Source: CAD feature listing. Evaluate the final solid. Frame: model axes, mm. A direction names the side the tool comes from. Round coordinates to 2 decimals unless told otherwise and drop trailing zeros. Order: outer loops, then holes, each group sorted by start corner. A loop starts at its lowest first (then second) coordinate and runs counter-clockwise, first axis right, second up. Notation, with made-up numbers: M 55.25,-4.75 L 78.25,-4.75 A24 ccw 78.25,29.25 Z; hole C -14,-18.75 d5. An arc over 180 degrees is marked long. Answer in a Markdown table with one row per item. Add a question column.
```python
from build123d import *

# Parameters (mm, degrees)
SKETCH1_W                 = 123
SKETCH1_H                 = 87.75
SKETCH1_W_2               = 113
SKETCH1_H_2               = 77.75
BOSS_EXTRUDE1_DEPTH       = 44
SKETCH1_3_W               = 113
SKETCH1_3_H               = 77.75
BOSS_EXTRUDE2_DEPTH       = 3
FILLET1_R                 = 15
FILLET2_R                 = 15
FILLET3_R                 = 15
FILLET4_R                 = 15
FILLET5_R                 = 15
FILLET6_R                 = 15
FILLET7_R                 = 15
FILLET8_R                 = 15
SKETCH2_R                 = 1.5
CUT_EXTRUDE1_DEPTH        = 116.837439975
LPATTERN2_COUNT           = 2
LPATTERN2_PITCH           = 32
LPATTERN2_COPY_1_SKETCH_R = 1.5
LPATTERN2_COPY_1_DEPTH    = 116.837439975
SKETCH3_R                 = 12.5
CUT_EXTRUDE2_DEPTH        = 138.804265627


with BuildPart() as part:
    # Sketch1 → Boss-Extrude1 (new body)
    with BuildSketch(Plane(origin=(0, 0, 0), x_dir=(1, 0, 0), z_dir=(0, 1, 0))):
        Rectangle(SKETCH1_W, SKETCH1_H)
        Rectangle(SKETCH1_W_2, SKETCH1_H_2, mode=Mode.SUBTRACT)
    extrude(amount=BOSS_EXTRUDE1_DEPTH)

    # Sketch1_3 → Boss-Extrude2 (add)
    with BuildSketch(Plane(origin=(0, 0, 0), x_dir=(1, 0, 0), z_dir=(0, 1, 0))):
        Rectangle(SKETCH1_3_W, SKETCH1_3_H)
    extrude(amount=BOSS_EXTRUDE2_DEPTH)

    # Fillet1
    fillet1_edges = [part.edges().sort_by_distance(p)[0] for p in [
        (-61.5, 22, 43.875),
    ]]
    fillet(fillet1_edges, radius=FILLET1_R)

    # Fillet2
    fillet2_edges = [part.edges().sort_by_distance(p)[0] for p in [
        (-61.5, 22, -43.875),
    ]]
    fillet(fillet2_edges, radius=FILLET2_R)

    # Fillet3
    fillet3_edges = [part.edges().sort_by_distance(p)[0] for p in [
        (61.5, 22, -43.875),
    ]]
    fillet(fillet3_edges, radius=FILLET3_R)

    # Fillet4
    fillet4_edges = [part.edges().sort_by_distance(p)[0] for p in [
        (61.5, 22, 43.875),
    ]]
    fillet(fillet4_edges, radius=FILLET4_R)

    # Fillet5
    fillet5_edges = [part.edges().sort_by_distance(p)[0] for p in [
        (-56.5, 23.5, -38.875),
    ]]
    fillet(fillet5_edges, radius=FILLET5_R)

    # Fillet6
    fillet6_edges = [part.edges().sort_by_distance(p)[0] for p in [
        (-56.5, 23.5, 38.875),
    ]]
    fillet(fillet6_edges, radius=FILLET6_R)

    # Fillet7
    fillet7_edges = [part.edges().sort_by_distance(p)[0] for p in [
        (56.5, 23.5, -38.875),
    ]]
    fillet(fillet7_edges, radius=FILLET7_R)

    # Fillet8
    fillet8_edges = [part.edges().sort_by_distance(p)[0] for p in [
        (56.5, 23.5, 38.875),
    ]]
    fillet(fillet8_edges, radius=FILLET8_R)

    # Sketch2 → Cut-Extrude1 (cut, through all)
    with BuildSketch(Plane(origin=(0, 0, -43.875), x_dir=(-1, 0, 0), z_dir=(0, 0, -1))):
        with Locations((-25.75, 6.25)):
            Circle(SKETCH2_R)
    cut_extrude1 = extrude(amount=-CUT_EXTRUDE1_DEPTH, mode=Mode.SUBTRACT)

    # Mirror1: Cut-Extrude1 across plane
    add(cut_extrude1.mirror(Plane(origin=(0, 0, 0), x_dir=(0, 0, 1), z_dir=(1, 0, 0))), mode=Mode.SUBTRACT)

    # LPattern2: Cut-Extrude1 ×2
    with Locations(*[(0, i * LPATTERN2_PITCH, 0) for i in range(1, LPATTERN2_COUNT)]):
        add(cut_extrude1, mode=Mode.SUBTRACT)

    # LPattern2 copy 1 sketch → LPattern2 copy 1 (cut, through all)
    with BuildSketch(Plane(origin=(0, 32, -43.875), x_dir=(1, 0, 0), z_dir=(0, 0, -1))):
        with Locations((-25.75, -6.25)):
            Circle(LPATTERN2_COPY_1_SKETCH_R)
    extrude(amount=-LPATTERN2_COPY_1_DEPTH, mode=Mode.SUBTRACT)

    # Sketch3 → Cut-Extrude2 (cut, through all)
    with BuildSketch(Plane.ZY.offset(61.5)):
        with Locations((0, 23.62)):
            Circle(SKETCH3_R)
    extrude(amount=-CUT_EXTRUDE2_DEPTH, mode=Mode.SUBTRACT)


solid = part.part
```
(1) Pin query (flat end, axial travel): pin 1 (1.5 mm diameter, centred on x = -24.5, z = 0.5, fed in from +Y). Return the tip coordinate at first contact, or that it passes through.
(2) Access query for faces 5 (the face through (56.989, 22.308, -39.598)), 6 (the face through (-1, 3, -1)). Directions: +Z, -Z, +X, -X, +Y, -Y. A direction counts if a zero-diameter tool reaches every point of the face in a straight line with its end or side. Return the directions, or none.
(3) Cut plane D-D (x = -4). Return loops of the section in (y, z) (3 decimals), and give its area (3 significant figures).
(4) Draft query along Y for faces 1 (the face through (27.25, 6.32, 41.34)), 2 (the face through (-27.25, 6.32, 41.34)), 3 (the face through (56.5, 37, 0)), 4 (the face through (-1, 0, -1)). Return one class per face: +Y half, -Y half, draft (parallel to the pull), parting line (faces both ways), or undercut.
(5) Cut plane A-A (z = 0). Return loops of the section in (x, y).
(6) Line query: line 1 (Y direction, x = 25.75, z = 42.7); line 2 (Z direction, x = 17, y = 34) (3 decimals); line 3 (X direction, y = 25, z = 19). Output: solid intervals per line, ascending. Write a range as from..to.
(7) Cut plane B-B (y = 38.25). Count the separate pieces of the cut face and the enclosed holes in it, and give its area (3 significant figures).
(8) Cut plane C-C (y = 23.62). Return loops of the section in (x, z) (3 decimals), and give its area (3 significant figures).
Answer list:
| question | item | result |
|---|---|---|
| 1 | pin 1 | y = 3 |
| 2 | face 5 | -Z, +X, +Y, -Y |
| 2 | face 6 | +Y |
| 3 | outline | M 0,-43.875 L 44,-43.875 L 44,-38.875 L 3,-38.875 L 3,38.875 L 44,38.875 L 44,43.875 L 0,43.875 Z |
| 3 | area | 673 mm² |
| 4 | face 1 | undercut |
| 4 | face 2 | undercut |
| 4 | face 3 | draft |
| 4 | face 4 | -Y half |
| 5 | outline | M -61.5,0 L 61.5,0 L 61.5,11.12 L 56.5,11.12 L 56.5,3 L -56.5,3 L -56.5,11.12 L -61.5,11.12 Z; M -61.5,36.12 L -56.5,36.12 L -56.5,44 L -61.5,44 Z; M 56.5,36.12 L 61.5,36.12 L 61.5,44 L 56.5,44 Z |
| 6 | line 1 | 0..4.75, 7.75..36.75, 39.75..44 |
| 6 | line 2 | -43.875..-38.875, 38.875..43.875 |
| 6 | line 3 | -61.5..-56.5, 56.5..61.5 |
| 7 | separate pieces | 4 |
| 7 | enclosed holes | 0 |
| 7 | area | 1,950 mm² |
| 8 | outline | M -61.5,-28.875 A15 ccw -46.5,-43.875 L 46.5,-43.875 A15 ccw 61.5,-28.875 L 61.5,-12.5 L 56.5,-12.5 L 56.5,-23.875 A15 cw 41.5,-38.875 L -41.5,-38.875 A15 cw -56.5,-23.875 L -56.5,-12.5 L -61.5,-12.5 Z; M -61.5,12.5 L -56.5,12.5 L -56.5,23.875 A15 cw -41.5,38.875 L 41.5,38.875 A15 cw 56.5,23.875 L 56.5,12.5 L 61.5,12.5 L 61.5,28.875 A15 ccw 46.5,43.875 L -46.5,43.875 A15 ccw -61.5,28.875 Z |
| 8 | area | 1,760 mm² |
